from build123d import *

# Parameters (mm, degrees)
F0_R     = 5.5
F0_R_2   = 3.6
F0_R_3   = 2.8
F1_DEPTH = 3
F2_DEPTH = 3
F3_R     = 1


with BuildPart() as f1:
    # F0 (on Top) → F1 (new body)
    with BuildSketch(Plane.XY):
        Circle(F0_R)
        Circle(F0_R_2, mode=Mode.SUBTRACT)
        Circle(F0_R_2)
        with Locations((0.072045, 0.007089)):
            Circle(F0_R_3, mode=Mode.SUBTRACT)
    extrude(amount=F1_DEPTH)

    # F0 (on Top) → F2 (join)
    with BuildSketch(Plane.XY):
        Circle(F0_R_2)
        with Locations((0.072045, 0.007089)):
            Circle(F0_R_3, mode=Mode.SUBTRACT)
    extrude(amount=-F2_DEPTH)

    # F3
    f3_edges = [f1.edges().sort_by_distance(p)[0] for p in [
        (-2.727955, 0.007089, 3),
        (-5.5, 0, 3),
    ]]
    fillet(f3_edges, radius=F3_R)


solid = f1.part
Could you check a few things on this model? Use its own coordinates, in mm. A direction names the side the tool comes from. Give positions to 0.01 mm unless a question says otherwise; leave off trailing zeros. Order: outer loops, then holes, each group sorted by start corner. A loop starts at its lowest first (then second) coordinate and runs counter-clockwise, first axis right, second up. Notation, with made-up numbers: (63, 68.25) - (119, 68.25) arc R36 ccw to (119, 105.25) - close; hole circle Ø2 at (-36.75, -28). An arc over 180 degrees is marked (long way). One line per question, with ' | ' between items. Start each with the question number.
Item 1: I want a section at A-A on z = -0.35. Write out the boundary of the cut face in (x, y), then the cut area to 3 significant figures.
Item 2: Thinking about a two-plate mould opening in Y: for faces 1 (the flat face through (-1, -3, -3)), 2 (the cylindrical face through (-0.535, -2.726, -0.535)), 3 (the cylindrical face through (3.434, 1.081, -1.479)), which applies, pulls with the +Y half, pulls with the -Y half, needs draft (parallel to the pull), parting line crosses it, or undercut?
Item 3: I need wall thicknesses on probe 1 along Y at (x, z) = (0, -1.15); probe 2 along Y at (x, z) = (0, 1.4); probe 3 along Z at (x, y) = (2, -3.5). Which ranges of each line are inside material? Lowest first, please. Write a range as [from, to].
Item 4: For faces 4 (the cylindrical face through (-1.19, -5.37, 0.99)), 5 (the flat face through (4, -1, 0)), which set-ups out of +Z, -Z, +X, -X, +Y, -Y let a thin tool reach every point of the face, with its end or its side?
Item 5: I'm going to push flat-ended pins straight in: pin 1 Ø2 at (y, z) = (-3.5, -1.5) entering from -X; pin 2 Ø1 at (y, z) = (0, -1) entering from -X; pin 3 Ø2 at (x, y) = (2.5, 4) entering from -Z. Where does each tip first touch, or does it pass through?
Verdict:
1) outline: circle Ø7.2 at (0, 0); hole circle Ø5.6 at (0.07, 0.01) | area: 16.1 mm^2
2) face 1: needs draft | face 2: undercut | face 3: parting line crosses it
3) probe 1: [-3.6, -2.79], [2.81, 3.6] | probe 2: [-5.5, -2.79], [2.81, 5.5] | probe 3: [0, 3]
4) face 4: +Z, -Z | face 5: -Z
5) pin 1: x = -2.59 | pin 2: x = -3.6 | pin 3: z = 0
